```python
from build123d import *


with BuildPart() as part:
    # Sketch1 → Revolve1 (revolve)
    with BuildSketch(Plane(origin=(0, 0, 0), x_dir=(1, 0, 0), z_dir=(0, 1, 0))):
        Polygon((-355, 76.3943727), (-355, 12.3), (-170, 12.716901408), (-170, 70.8239497), align=None)
        Polygon((-170, 70.8239497), (-170, 12.716901408), (-119, 12.831830986), (-119, 68.7549354), align=None)
        with BuildLine():
            Line((-119, 68.7549354), (-119, 12.831830986))
            Line((-119, 12.831830986), (0, 13.1))
            ThreePointArc((0, 13.1), (-53.314248435, 54.153687996), (-119, 68.7549354))
        make_face()
    revolve(axis=Axis((-69.290541893, 0, 0), (1, 0, 0)))


solid = part.part
```
Check sheet for the modelled part. Datum: model origin and axes. Units: mm. A direction names the side the tool comes from. Round coordinates to 2 decimals unless told otherwise and drop trailing zeros. Order: outer loops, then holes, each group sorted by start corner. A loop starts at its lowest first (then second) coordinate and runs counter-clockwise, first axis right, second up. Notation, with made-up numbers: (24.25, 29.5) - (56.25, 29.5) arc R9 ccw to (56.25, 44.5) - close; hole circle Ø7 at (25.5, 45). An arc over 180 degrees is marked (long way). Answer as CSV lines item,"result". Start each with the question number.
1) Tool access check on faces 1 (the face through (-355, 1, -16)), 2 (the face through (-263.8, 22.12, -70.25)). Record the directions out of +Z, -Z, +X, -X, +Y, -Y that give a thin tool (end or side, any length) a straight path to the whole face; none if there is none.
2) Section check A-A (x = -250). Record the cut outline in (y, z), then the cut area to 3 significant figures.
3) Section check B-B (x = -177). Record the cut outline in (y, z).
4) Scan lines: probe 1 along Y at (x, z) = (-337, 8.5); probe 2 along Y at (x, z) = (-141, -0.5); probe 3 along Z at (x, y) = (-285.5, 3). Record each from-to range of solid material in increasing order.
5) Depth check by flat-ended pin: pin 1 (4 mm diameter, centred on x = -134.5, y = 43.5, fed in from +Z); pin 2 (6 mm diameter, centred on x = -180, y = -38, fed in from +Z); pin 3 (6 mm diameter, centred on y = 38.5, z = 2.5, fed in from +X). Enter the tip coordinate at first touch or a pass-through.
Determined:
1,face 1,"+Z, -Z, -X, +Y, -Y"
1,face 2,"+X"
2,outline,"circle Ø146.47 at (0, 0); hole circle Ø25.07 at (0, 0)"
2,area,"16,400 mm^2"
3,outline,"circle Ø142.07 at (0, 0); hole circle Ø25.4 at (0, 0)"
4,probe 1,"-75.37 to -8.95, 8.95 to 75.37"
4,probe 2,"-69.65 to -12.77, 12.77 to 69.65"
4,probe 3,"-74.24 to -12.09, 12.09 to 74.24"
5,pin 1,"z = 55.61"
5,pin 2,"z = 61.92"
5,pin 3,"x = -23.15"
